Here's how the part is built. I have some questions about the finished solid (model axes, mm). A direction names the side the tool comes from. Coordinates: 2 decimals unless noted, no trailing zeros. Write each loop counter-clockwise with the first axis right and the second up, starting at its lowest first coordinate (ties: lowest second). Pieces come first, ordered by that corner, then holes. Notation, with made-up numbers: (9, 64) - (33, 64) arc R17 cw to (33, 88) - close; hole circle Ø8 at (83, 21). An arc over 180 degrees is marked (long way). Answer in a Markdown table with one row per item. Add a question column.
Item 1: If I drill on probe 1 along Y at (x, z) = (15.76, -0.6); probe 2 along X at (y, z) = (-24.5, -1.45), over which ranges is the centre line in solid material (lowest first)? Write a range as from..to.
Item 2: We'd pull the mould along X, two halves only. Please class faces 1 (the face through (15.542, -1.521, -26.018)), 2 (the face through (28, 0, -14)), 3 (the face through (48.51, -14, -23)): +X half, -X half, draft (parallel to the pull), parting line (faces both ways), or undercut.
Item 3: Imagine slicing it at A-A (z = -1.75). Please give me the cut outline in (x, y), plus the area to 3 significant figures.
Item 4: I'm going to push flat-ended pins straight in: pin 1 (3 mm diameter, centred on x = 6, y = -3, fed in from -Z); pin 2 (4 mm diameter, centred on x = 46, z = -22.5, fed in from -Y) (3 decimals); pin 3 (1 mm diameter, centred on y = -7.5, z = -10.5, fed in from +X). Where does each tip first touch, or does it pass through?
Item 5: Imagine slicing it at D-D (z = -10.25). Please give me the cut outline in (x, y).
Item 6: Imagine slicing it at B-B (x = 5). Please give me the cut outline in (y, z).
Item 7: Imagine slicing it at C-C (y = -9.5). Please give me the cut outline in (x, z).
Item 8: Which directions (+Z, -Z, +X, -X, +Y, -Y) give clear straight access to the entire face, cutting with the end or side of a thin tool? Please do faces 4 (the face through (13.51, -3, -4)), 5 (the face through (14.792, -22.982, -1.521)), 6 (the face through (46, -3.725, -23)), 7 (the face through (16.744, -1.521, -6.285)), 8 (the face through (46, -15, -18.5)).
from build123d import *

# Parameters (mm, degrees)
SKETCH1_W                = 29
SKETCH1_H                = 29
BOSS_EXTRUDE1_DEPTH      = 48.51
CUT_EXTRUDE1_DEPTH       = 13.51
M3_CLEARANCE_HOLE3_D     = 3.6
M3_CLEARANCE_HOLE3_DEPTH = 3
M3_CLEARANCE_HOLE3_TIP   = 1.081549114
SKETCH6_W                = 29
SKETCH6_H                = 29
SKETCH6_W_2              = 8.5
SKETCH6_H_2              = 21.55
CUT_EXTRUDE2_DEPTH       = 5
M3_CLEARANCE_HOLE2_D     = 3.6
M3_CLEARANCE_HOLE2_DEPTH = 3
M3_CLEARANCE_HOLE2_TIP   = 1.081549114


with BuildPart() as part:
    # Sketch1 → Boss-Extrude1 (new body)
    with BuildSketch(Plane(origin=(0, 0, 0), x_dir=(0, -1, 0), z_dir=(1, 0, 0))):
        with Locations((14.5, 14.5)):
            Rectangle(SKETCH1_W, SKETCH1_H)
    extrude(amount=BOSS_EXTRUDE1_DEPTH)

    # Sketch2 → Cut-Extrude1 (cut)
    with BuildSketch(Plane.ZY):
        with BuildLine():
            Line((-14.500000026, 0), (-29, 0))
            Line((-29, 0), (-24.753048327, -4.246951673))
            ThreePointArc((-24.753048327, -4.246951673), (-20.048909781, -1.103746784), (-14.500000026, 0))
        make_face()
        with BuildLine():
            Line((-24.753048327, -4.246951673), (-29, 0))
            Line((-29, 0), (-29, -14.499999948))
            ThreePointArc((-29, -14.499999948), (-27.896253211, -8.951090207), (-24.753048327, -4.246951673))
        make_face()
        with BuildLine():
            ThreePointArc((-14.5, -29), (-24.753048346, -24.753048309), (-29, -14.499999948))
            Line((-29, -14.499999948), (-29, -29))
            Line((-29, -29), (-14.5, -29))
        make_face()
        with BuildLine():
            Line((0, -29), (-4.246951673, -24.753048327))
            ThreePointArc((-4.246951673, -24.753048327), (-8.951090231, -27.896253221), (-14.5, -29))
            Line((-14.5, -29), (0, -29))
        make_face()
        with BuildLine():
            ThreePointArc((0, -14.5), (-1.103746779, -20.048909769), (-4.246951673, -24.753048327))
            Line((-4.246951673, -24.753048327), (0, -29))
            Line((0, -29), (0, -14.5))
        make_face()
        with BuildLine():
            Line((0, 0), (-14.500000026, 0))
            ThreePointArc((-14.500000026, 0), (-4.246951682, -4.246951664), (0, -14.5))
            Line((0, -14.5), (0, 0))
        make_face()
    extrude(amount=-CUT_EXTRUDE1_DEPTH, mode=Mode.SUBTRACT)

    # M3 Clearance Hole3
    with Locations(Plane.XY):
        with Locations((15.76, -24.5), (15.76, -4.5)):
            Hole(M3_CLEARANCE_HOLE3_D / 2, depth=M3_CLEARANCE_HOLE3_DEPTH)
            with Locations((0, 0, -(M3_CLEARANCE_HOLE3_DEPTH + M3_CLEARANCE_HOLE3_TIP / 2))):  # 118° drill point
                Cone(0, M3_CLEARANCE_HOLE3_D / 2, M3_CLEARANCE_HOLE3_TIP, mode=Mode.SUBTRACT)

    # Sketch6 → Cut-Extrude2 (cut)
    with BuildSketch(Plane(origin=(48.51, 0, 0), x_dir=(0, 0, -1), z_dir=(1, 0, 0))):
        with Locations((14.5, -14.5)):
            Rectangle(SKETCH6_W, SKETCH6_H)
        with Locations((22.75, -14.5)):
            Rectangle(SKETCH6_W_2, SKETCH6_H_2, mode=Mode.SUBTRACT)
    extrude(amount=-CUT_EXTRUDE2_DEPTH, mode=Mode.SUBTRACT)

    # M3 Clearance Hole2
    with Locations(Plane(origin=(0, 0, 0), x_dir=(1, 0, 0), z_dir=(0, 1, 0))):
        with Locations((16.51, 24.5), (16.51, 4.5), (40.21, 14.5)):
            Hole(M3_CLEARANCE_HOLE2_D / 2, depth=M3_CLEARANCE_HOLE2_DEPTH)
            with Locations((0, 0, -(M3_CLEARANCE_HOLE2_DEPTH + M3_CLEARANCE_HOLE2_TIP / 2))):  # 118° drill point
                Cone(0, M3_CLEARANCE_HOLE2_D / 2, M3_CLEARANCE_HOLE2_TIP, mode=Mode.SUBTRACT)


solid = part.part
Here are the results:
| question | item | result |
|---|---|---|
| 1 | probe 1 | y = -29..-26.3, -22.7..-6.3, -2.7..0 |
| 1 | probe 2 | x = 13.51..13.96, 17.56..43.51 |
| 2 | face 1 | undercut |
| 2 | face 2 | draft |
| 2 | face 3 | +X half |
| 3 | outline | (0, -21.41) - (13.51, -21.41) - (13.51, -29) - (43.51, -29) - (43.51, 0) - (13.51, 0) - (13.51, -7.59) - (0, -7.59) - close; hole circle Ø3.6 at (15.76, -24.5); hole circle Ø3.6 at (15.76, -4.5) |
| 3 | area | 1,040 mm2 |
| 4 | pin 1 | stops at z = -25 |
| 4 | pin 2 | stops at y = -25.275 |
| 4 | pin 3 | stops at x = 43.51 |
| 5 | outline | (0, -28.36) - (13.51, -28.36) - (13.51, -29) - (43.51, -29) - (43.51, 0) - (13.51, 0) - (13.51, -0.64) - (0, -0.64) - close |
| 6 | outline | circle Ø29 at (-14.5, -14.5) |
| 7 | outline | (0, -28.11) - (13.51, -28.11) - (13.51, -29) - (43.51, -29) - (43.51, -27) - (48.51, -27) - (48.51, -18.5) - (43.51, -18.5) - (43.51, 0) - (13.51, 0) - (13.51, -0.89) - (0, -0.89) - close |
| 8 | face 4 | +Z, -X, +Y |
| 8 | face 5 | +Z |
| 8 | face 6 | +Z, -Z, +X, +Y |
| 8 | face 7 | +Y |
| 8 | face 8 | +Z, +X, +Y, -Y |
